Build history of the part. All positions in model axes, mm. Give positions to 0.01 mm unless a question says otherwise; leave off trailing zeros. Loops run counter-clockwise (first coordinate to the right, second up) from the corner with the lowest first, then second, coordinate; pieces in that order, holes last. Notation, with made-up numbers: M -32,-19.75 L -27,-19.75 A31 cw -27,4.25 Z; hole C -21.75,2.5 d8. An arc over 180 degrees is marked long. Put each result on its own line as item: value.
Autodesk Inventor part; units mm, degrees
ref_plane "YZ Plane" through (0, 0, 0) normal (1, 0, 0) x (0, 1, 0)
ref_plane "XZ Plane" through (0, 0, 0) normal (0, 1, 0) x (-1, 0, 0)
ref_plane "XY Plane" through (0, 0, 0) normal (0, 0, 1) x (1, 0, 0)
sketch "Sketch1" plane through (0, 0, 0) normal (0, 0, 1) x (1, 0, 0)
  line L0 (0, 0) -> (600, 0)
  line L1 (600, 0) -> (600, 89)
  line L2 (600, 89) -> (0, 89)
  line L3 (0, 89) -> (0, 0)
  line L4 (105, 0) -> (145, 0)
  line L5 (145, 0) -> (145, -5.5)
  line L6 (145, -5.5) -> (105, -5.5)
  line L7 (105, -5.5) -> (105, 0)
  line L8 (280, 0) -> (320, 0)
  line L9 (320, 0) -> (320, -5.5)
  line L10 (320, -5.5) -> (280, -5.5)
  line L11 (280, -5.5) -> (280, 0)
  line L12 (480, 0) -> (520, 0)
  line L13 (520, 0) -> (520, -5.5)
  line L14 (520, -5.5) -> (480, -5.5)
  line L15 (480, -5.5) -> (480, 0)
  line L16 (105, 89) -> (145, 89)
  line L17 (145, 89) -> (145, 94.5)
  line L18 (145, 94.5) -> (105, 94.5)
  line L19 (105, 94.5) -> (105, 89)
  line L20 (280, 89) -> (320, 89)
  line L21 (320, 89) -> (320, 94.5)
  line L22 (320, 94.5) -> (280, 94.5)
  line L23 (280, 94.5) -> (280, 89)
  line L24 (480, 89) -> (520, 89)
  line L25 (520, 89) -> (520, 94.5)
  line L26 (520, 94.5) -> (480, 94.5)
  line L27 (480, 94.5) -> (480, 89)
  line L28 (0, 24.5) -> (5.5, 24.5)
  line L29 (5.5, 24.5) -> (5.5, 64.5)
  line L30 (5.5, 64.5) -> (0, 64.5)
  line L31 (0, 64.5) -> (0, 24.5)
  line L32 (600, 24.5) -> (594.5, 24.5)
  line L33 (594.5, 24.5) -> (594.5, 64.5)
  line L34 (594.5, 64.5) -> (600, 64.5)
  line L35 (600, 64.5) -> (600, 24.5)
  dimension "d0" = 600
  dimension "d1" = 89
  dimension "d2" = 40
  dimension "d3" = 5.5
  dimension "d4" = 40
  dimension "d5" = 5.5
  dimension "d6" = 40
  dimension "d7" = 5.5
  dimension "d8" = 5.5
  dimension "d9" = 40
  dimension "d10" = 5.5
  dimension "d11" = 40
extrude "Extrusion1" add sketch "Sketch1" along normal blind 5.5 contours L3 L28 L29 L30 L2 L1 L34 L33 L32 L0 | L0 L5 L6 L7 | L0 L9 L10 L11 | L19 L18 L17 L2 | L0 L13 L14 L15 | L23 L22 L21 L2 | L27 L26 L25 L2
properties part number "techo"
Q1. Drop flat-ended pins along their axis: pin 1 Ø3 at (y, z) = (92.5, 3.5) entering from +X; pin 2 Ø1 at (y, z) = (38, 2.5) entering from -X; pin 3 Ø3 at (y, z) = (58, 2) entering from +X. Give the stop position or say it passes through.
Here are the results:
pin 1: x = 520
pin 2: x = 5.5
pin 3: x = 594.5
Q2. Slice it at A-A (x = 344). List the corners of the cut face in (y, z), and give its area (4 significant figures).
Here are the results:
outline: M 0,0 L 89,0 L 89,5.5 L 0,5.5 Z
area: 489.5 mm²
Q3. Probe line 1 (X direction, y = 44, z = 4.7); line 2 (Y direction, x = 410, z = 0.5). List the from-to ranges inside material, lowest first. Write a range as from..to.
Here are the results:
line 1: 5.5..594.5
line 2: 0..89
Q4. Slice it at B-B (y = 56.5). List the corners of the cut face in (x, z).
Here are the results:
outline: M 5.5,0 L 594.5,0 L 594.5,5.5 L 5.5,5.5 Z
